CAD build for the part. Positions are in the model's coordinates, mm. Face numbers are marked on the shaded views. A direction names the side the tool comes from. Coordinates: 2 decimals unless noted, no trailing zeros. Order: outer loops, then holes, each group sorted by start corner. A loop starts at its lowest first (then second) coordinate and runs counter-clockwise, first axis right, second up. Notation, with made-up numbers: M 40,32 L 63,32 A29 cw 63,60 Z; hole C 18.5,8 d11. An arc over 180 degrees is marked long. One line per item, written item: value.
from build123d import *

# Parameters (mm, degrees)
SKETCH1_W           = 50.165
SKETCH1_H           = 15.875
SKETCH1_R           = 3.302
BOSS_EXTRUDE1_DEPTH = 6.35
BOSS_EXTRUDE2_DEPTH = 15.875
FILLET1_R           = 6.35
SKETCH1_3_R         = 3.302
CUT_EXTRUDE1_DEPTH  = 47.300601643
SKETCH10_R          = 5.08
CUT_EXTRUDE4_DEPTH  = 42.233459866


with BuildPart() as part:
    # Sketch1 → Boss-Extrude1 (new body)
    with BuildSketch(Plane.XY):
        Rectangle(SKETCH1_W, SKETCH1_H)
        with Locations((5.23875, 0)):
            Circle(SKETCH1_R, mode=Mode.SUBTRACT)
        with Locations((-10.63625, 0)):
            Circle(SKETCH1_R, mode=Mode.SUBTRACT)
    extrude(amount=BOSS_EXTRUDE1_DEPTH)

    # Sketch4 → Boss-Extrude2 (add, through all)
    with BuildSketch(Plane.XZ.offset(7.9375)):
        with BuildLine():
            Line((-25.0825, 6.35), (25.0825, 6.35))
            Line((25.0825, 6.35), (25.0825, 8.382))
            ThreePointArc((25.0825, 8.382), (15.884529206, 19.05), (25.0825, 29.718))
            Line((25.0825, 29.718), (25.0825, 38.1))
            Line((25.0825, 38.1), (-25.0825, 6.35))
        make_face()
    extrude(amount=-BOSS_EXTRUDE2_DEPTH)

    # Fillet1
    fillet1_edges = [part.edges().sort_by_distance(p)[0] for p in [
        (25.0825, 0, 8.382),
        (25.0825, 0, 29.718),
    ]]
    fillet(fillet1_edges, radius=FILLET1_R)

    # Sketch1<3> → Cut-Extrude1 (cut, through all)
    with BuildSketch(Plane.XY):
        with Locations(Location((5.23875, 0, 0), (0, 0, 180))):
            Circle(SKETCH1_3_R)
        with Locations(Location((-10.63625, 0, 0), (0, 0, 180))):
            Circle(SKETCH1_3_R)
    extrude(amount=CUT_EXTRUDE1_DEPTH, mode=Mode.SUBTRACT)

    # Sketch10 → Cut-Extrude4 (cut, through all)
    with BuildSketch(Plane(origin=(0, 0, 6.35), x_dir=(-1, 0, 0), z_dir=(0, 0, -1))):
        with Locations((10.63625, 0)):
            Circle(SKETCH10_R)
        with Locations((-5.23875, 0)):
            Circle(SKETCH10_R)
    extrude(amount=-CUT_EXTRUDE4_DEPTH, mode=Mode.SUBTRACT)


solid = part.part
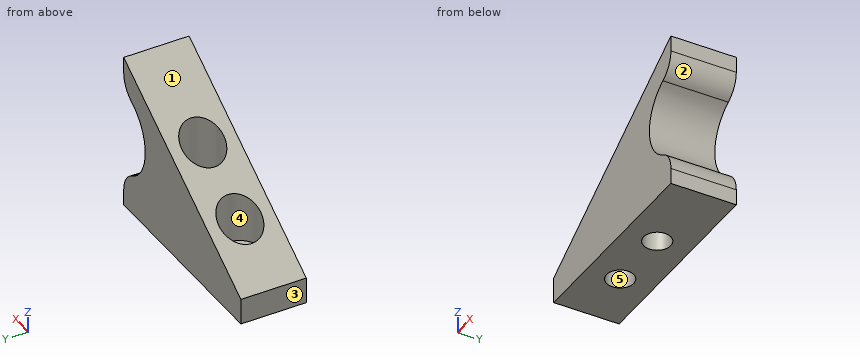
Q1. Drill centre lines: line 1 along X through (y, z) = (0, 11.75); line 2 along X through (y, z) = (1.5, 5); line 3 along Z through (x, y) = (17, -4.5). Where is each one in solid material? Low to high.
Recorded:
line 1: x = -16.55 to -15.72, -5.56 to 0.16, 10.32 to 18.73
line 2: x = -25.08 to -13.58, -7.69 to 2.3, 8.18 to 24.98
line 3: z = 0 to 14.27, 23.83 to 32.98
Q2. Slice it at A-A (x = 2.5). List the corners of the cut face in (y, z), plus the area to 3 significant figures.
Recorded:
outline: M -7.94,0 L -1.84,0 L -1.84,6.35 L -4.28,6.35 L -4.28,23.81 L -7.94,23.81 Z; M 1.84,0 L 7.94,0 L 7.94,23.81 L 4.28,23.81 L 4.28,6.35 L 1.84,6.35 Z
area: 205 mm^2
Q3. Slice it at D-D (y = 4.5). List the corners of the cut face in (x, z), plus the area to 3 significant figures.
Recorded:
outline: M -25.08,0 L 25.08,0 L 25.08,3.86 A6.35 ccw 21.67,9.49 A10.79 cw 21.67,28.61 A6.35 ccw 25.08,34.24 L 25.08,38.1 L 7.6,27.03 L 7.6,6.35 L 2.88,6.35 L 2.88,24.05 L -8.28,16.99 L -8.28,6.35 L -12.99,6.35 L -12.99,14 L -25.08,6.35 Z
area: 826 mm^2
Q4. Mould opens along Z. For the marked faces 1, 2 and 3 say: released by +Z, released by -Z, zero draft, split by the parting line, or undercut.
Recorded:
face 1: released by +Z
face 2: undercut
face 3: zero draft
Q5. Slice it at C-C (y = 0). List the corners of the cut face in (x, z).
Recorded:
outline: M -25.08,0 L -13.94,0 L -13.94,6.35 L -15.72,6.35 L -15.72,12.28 L -25.08,6.35 Z; M -7.33,0 L 1.94,0 L 1.94,6.35 L 0.16,6.35 L 0.16,22.33 L -5.56,18.71 L -5.56,6.35 L -7.33,6.35 Z; M 8.54,0 L 25.08,0 L 25.08,3.86 A6.35 ccw 21.67,9.49 A10.79 cw 21.67,28.61 A6.35 ccw 25.08,34.24 L 25.08,38.1 L 10.32,28.76 L 10.32,6.35 L 8.54,6.35 Z
Q6. Which spindle directions (+Z, -Z, +X, -X, +Y, -Y) get a long thin tool onto all of the face, cutting with end or side? Do the marked faces 4 and 5. Say none if no direction does.
Recorded:
face 4: +Z
face 5: +Z, -Z
Q7. Pin check, flat tips, straight feed: pin 1 Ø6 at (x, y) = (5.24, 0) entering from -Z; pin 2 Ø8 at (x, y) = (-10.64, 0) entering from +Z; pin 3 Ø8 at (x, y) = (13, -4.5) entering from +Z; pin 4 Ø6 at (x, y) = (6, 2.5) entering from +Z. Stop position of each tip, or through.
Recorded:
pin 1: passes through
pin 2: stops at z = 6.35
pin 3: stops at z = 32.98
pin 4: stops at z = 27.78
Q8. Slice it at B-B (z = 16). List the corners of the cut face in (x, y), plus the area to 3 significant figures.
Recorded:
outline: M -9.84,-7.94 L 16.32,-7.94 L 16.32,7.94 L -9.84,7.94 L -9.84,5.02 A5.08 cw -9.84,-5.02 Z; hole C 5.24,0 d10.16
area: 302 mm^2
